from build123d import *

# Parameters (mm, degrees)
SALIENTE_EXTRUIR1_DEPTH = 1
CROQUIS2_W              = 82
CROQUIS2_H              = 1
SALIENTE_EXTRUIR2_DEPTH = 1.5
CROQUIS3_W              = 1
CROQUIS3_H              = 82
SALIENTE_EXTRUIR3_DEPTH = 1.5
CROQUIS4_W              = 82
CROQUIS4_H              = 1
SALIENTE_EXTRUIR4_DEPTH = 1.5
CROQUIS5_W              = 1
CROQUIS5_H              = 82
SALIENTE_EXTRUIR5_DEPTH = 1.5
CORTAR_EXTRUIR1_DEPTH   = 105.271280802
REDONDEO1_R             = 0.1
REDONDEO2_R             = 1.1


with BuildPart() as part:
    # Croquis1 → Saliente-Extruir1 (new body)
    with BuildSketch(Plane.XZ.offset(-44.742417107)):
        with BuildLine():
            Line((20, -96), (20, -6))
            ThreePointArc((20, -6), (14, 0), (8, -6))
            Line((8, -6), (8, -96))
            ThreePointArc((8, -96), (14, -102), (20, -96))
        make_face()
    extrude(amount=-SALIENTE_EXTRUIR1_DEPTH)

    # Croquis2 → Saliente-Extruir2 (add)
    with BuildSketch(Plane(origin=(20, 0, 0), x_dir=(0, 0, -1), z_dir=(1, 0, 0))):
        with Locations((51, 45.242417107)):
            Rectangle(CROQUIS2_W, CROQUIS2_H)
    extrude(amount=SALIENTE_EXTRUIR2_DEPTH)

    # Croquis3 → Saliente-Extruir3 (add)
    with BuildSketch(Plane.XZ.offset(-44.742417107)):
        with Locations((21, -51)):
            Rectangle(CROQUIS3_W, CROQUIS3_H)
    extrude(amount=SALIENTE_EXTRUIR3_DEPTH)

    # Croquis4 → Saliente-Extruir4 (add)
    with BuildSketch(Plane.ZY.offset(-8)):
        with Locations((-51, 45.242417107)):
            Rectangle(CROQUIS4_W, CROQUIS4_H)
    extrude(amount=SALIENTE_EXTRUIR4_DEPTH)

    # Croquis5 → Saliente-Extruir5 (add)
    with BuildSketch(Plane.XZ.offset(-44.742417107)):
        with Locations((7, -51)):
            Rectangle(CROQUIS5_W, CROQUIS5_H)
    extrude(amount=SALIENTE_EXTRUIR5_DEPTH)

    # Croquis6 → Cortar-Extruir1 (cut, through all)
    with BuildSketch(Plane(origin=(0, 45.742417107, 0), x_dir=(-1, 0, 0), z_dir=(0, 1, 0))):
        with BuildLine():
            Line((-12, -84), (-12, -18))
            ThreePointArc((-12, -18), (-14, -16), (-16, -18))
            Line((-16, -18), (-16, -84))
            ThreePointArc((-16, -84), (-14, -86), (-12, -84))
        make_face()
    extrude(amount=-CORTAR_EXTRUIR1_DEPTH, mode=Mode.SUBTRACT)

    # Redondeo1
    redondeo1_edges = [part.edges().sort_by_distance(p)[0] for p in [
        (20.5, 44.742417107, -51),
        (7.5, 44.742417107, -51),
    ]]
    fillet(redondeo1_edges, radius=REDONDEO1_R)

    # Redondeo2
    redondeo2_edges = [part.edges().sort_by_distance(p)[0] for p in [
        (21.5, 45.742417107, -51),
        (6.5, 45.742417107, -51),
    ]]
    fillet(redondeo2_edges, radius=REDONDEO2_R)


solid = part.part
Check sheet for the modelled part. Datum: model origin and axes. Units: mm. Give positions to 0.01 mm unless a question says otherwise; leave off trailing zeros. Loops run counter-clockwise (first coordinate to the right, second up) from the corner with the lowest first, then second, coordinate; pieces in that order, holes last. Notation, with made-up numbers: M 72,-40 L 107,-40 A30 ccw 107,-12 Z; hole C -24.75,68.5 d2. An arc over 180 degrees is marked long. Use a Markdown table: item, result. Add a question column.
Q1. Scan lines: line 1 along X through (y, z) = (43.6, -34); line 2 along X through (y, z) = (45.45, -96); line 3 along Y through (x, z) = (9.25, -51). Record each from-to range of solid material in increasing order. Write a range as [from, to].
Q2. Sectioned sample at B-B, the plane y = 43.7. Record the cut outline in (x, z), then the cut area to 3 significant figures.
Q3. Go/stop test with flat-tipped pins: pin 1 (0.5 mm diameter, centred on y = 45, z = -7.5, fed in from +X); pin 2 (0.8 mm diameter, centred on x = 21, y = 44.5, fed in from +Z); pin 3 (0.5 mm diameter, centred on y = 45.5, z = -94, fed in from -X). Record where each tip stops, or that it passes through.
Q4. Sectioned sample at C-C, the plane x = 15. Record the cut outline in (y, z), then the cut area to 3 significant figures.
Q5. Sectioned sample at D-D, the plane z = -89.5. Record the cut outline in (x, y).
Q6. Sectioned sample at A-A, the plane z = -53.5. Record the cut outline in (x, y).
Q7. Mould release check, pull along Z, two halves, no side actions. Record for faces 1 (the cylindrical face through (14, 45, -16)), 2 (the flat face through (11, 44.742, -50)), 3 (the cylindrical face through (14, 45, -86)), 4 (the cylindrical face through (14, 45, -102)): pulls with the +Z half, pulls with the -Z half, needs draft (parallel to the pull), parting line crosses it, or undercut.
Verdict:
| question | item | result |
|---|---|---|
| 1 | line 1 | [6.5, 7.5], [20.5, 21.5] |
| 1 | line 2 | [8, 20] |
| 1 | line 3 | [44.74, 45.74] |
| 2 | outline | M 6.5,-92 L 7.5,-92 L 7.5,-10 L 6.5,-10 Z; M 20.5,-92 L 21.5,-92 L 21.5,-10 L 20.5,-10 Z |
| 2 | area | 164 mm^2 |
| 3 | pin 1 | x = 20 |
| 3 | pin 2 | z = -10 |
| 3 | pin 3 | x = 8 |
| 4 | outline | M 44.74,-101.92 L 45.74,-101.92 L 45.74,-85.73 L 44.74,-85.73 Z; M 44.74,-16.27 L 45.74,-16.27 L 45.74,-0.08 L 44.74,-0.08 Z |
| 4 | area | 32.4 mm^2 |
| 5 | outline | M 6.5,43.24 L 7.5,43.24 L 7.5,44.64 A0.1 cw 7.6,44.74 L 20.4,44.74 A0.1 cw 20.5,44.64 L 20.5,43.24 L 21.5,43.24 L 21.5,44.64 A1.1 ccw 20.4,45.74 L 7.6,45.74 A1.1 ccw 6.5,44.64 Z |
| 6 | outline | M 6.5,43.24 L 7.5,43.24 L 7.5,44.64 A0.1 cw 7.6,44.74 L 12,44.74 L 12,45.74 L 7.6,45.74 A1.1 ccw 6.5,44.64 Z; M 16,44.74 L 20.4,44.74 A0.1 cw 20.5,44.64 L 20.5,43.24 L 21.5,43.24 L 21.5,44.64 A1.1 ccw 20.4,45.74 L 16,45.74 Z |
| 7 | face 1 | undercut |
| 7 | face 2 | needs draft |
| 7 | face 3 | undercut |
| 7 | face 4 | pulls with the -Z half |
